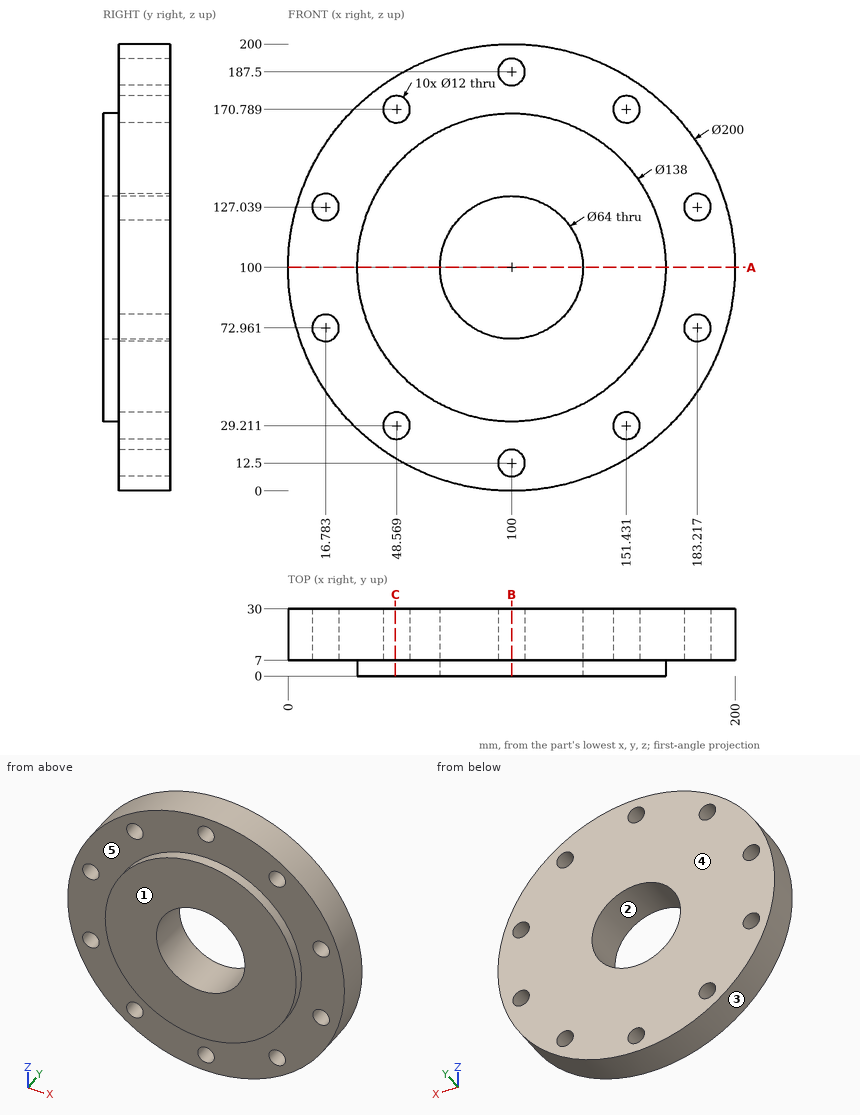
Part print with two shaded views. Sizes in mm from the minimum x, y, z corner. A direction names the side the tool comes from. Round coordinates to 2 decimals unless told otherwise and drop trailing zeros. Order: outer loops, then holes, each group sorted by start corner. A loop starts at its lowest first (then second) coordinate and runs counter-clockwise, first axis right, second up. Notation, with made-up numbers: M 29,83.5 L 33,83.5 A18 cw 33,88.5 Z; hole C 54,-32 d5. An arc over 180 degrees is marked long. Answer in a Markdown table with one row per item. Add a question column.
Q1. Mould opens along Z. For the marked faces 1, 2 and 3 say: +Z half, -Z half, draft (parallel to the pull), parting line (faces both ways), or undercut.
Q2. Cut at A-A on z = 100. Give the cut face in (x, y), and give its area (3 significant figures).
Q3. Cut at B-B on x = 100. Give the cut face in (y, z).
Q4. Wall check: L1, parallel to Z at x = 95, y = 27.75 (1 decimal); L2, parallel to X at y = 27.5, z = 72.5 (1 decimal); L3, parallel to X at y = 20.25, z = 166 (1 decimal). Give the ranges that are in metal, low to high. Write a range as from..to.
Q5. Cut at C-C on x = 48. Give the cut face in (y, z) (1 decimal).
Q6. 3-axis set-ups, long thin cutter, end or side, ignore diameter. For the marked faces 4 and 5: which of +Z, -Z, +X, -X, +Y, -Y reach the whole face in a straight line?
Q7. Pin check, flat tips, straight feed: pin 1 (7 mm diameter, centred on x = 100, z = 12.5, fed in from +Y); pin 2 (6 mm diameter, centred on x = 76.5, y = 18.5, fed in from -Z); pin 3 (15.5 mm diameter, centred on x = 183.22, z = 72.96, fed in from -Y); pin 4 (4 mm diameter, centred on y = 19.5, z = 45.5, fed in from -X). Stop position of each tip, or through.
Established:
| question | item | result |
|---|---|---|
| 1 | face 1 | draft |
| 1 | face 2 | undercut |
| 1 | face 3 | parting line |
| 2 | outline | M 0,7 L 31,7 L 31,0 L 68,0 L 68,30 L 0,30 Z; M 132,0 L 169,0 L 169,7 L 200,7 L 200,30 L 132,30 Z |
| 2 | area | 3,650 mm2 |
| 3 | outline | M 0,31 L 7,31 L 7,18.5 L 30,18.5 L 30,68 L 0,68 Z; M 0,132 L 30,132 L 30,181.5 L 7,181.5 L 7,169 L 0,169 Z; M 7,0 L 30,0 L 30,6.5 L 7,6.5 Z; M 7,193.5 L 30,193.5 L 30,200 L 7,200 Z |
| 4 | L1 | z = 0.1..9.2, 15.8..68.4, 131.6..184.2, 190.8..199.9 |
| 4 | L2 | x = 3.9..10.8, 22.8..83.6, 116.4..177.2, 189.2..196.1 |
| 4 | L3 | x = 24.9..45, 52.2..147.8, 155..175.1 |
| 5 | outline | M 0,54.6 L 7,54.6 L 7,35.2 L 30,35.2 L 30,164.8 L 7,164.8 L 7,145.4 L 0,145.4 Z; M 7,14.6 L 30,14.6 L 30,23.2 L 7,23.2 Z; M 7,176.8 L 30,176.8 L 30,185.4 L 7,185.4 Z |
| 6 | face 4 | +Z, -Z, +X, -X, +Y |
| 6 | face 5 | -Y |
| 7 | pin 1 | passes through |
| 7 | pin 2 | stops at z = 2.12 |
| 7 | pin 3 | stops at y = 7 |
| 7 | pin 4 | stops at x = 14.89 |
